Model file for the job. Use its own axes, mm. Face numbers are marked on the shaded views. A direction names the side the tool comes from. Give positions to 0.01 mm unless a question says otherwise; leave off trailing zeros. Write each loop counter-clockwise with the first axis right and the second up, starting at its lowest first coordinate (ties: lowest second). Pieces come first, ordered by that corner, then holes. Notation, with made-up numbers: (-29.75, 26.5) - (14.25, 26.5) arc R16 cw to (14.25, 33.5) - close; hole circle Ø11 at (-1.5, 85). An arc over 180 degrees is marked (long way). One line per item, written item: value. Start each with the question number.
(1) Cut at A-A, the plane y = -1.25. List the corners of the cut face in (x, z).
(2) Cut at D-D, the plane x = 0. List the corners of the cut face in (y, z), and give its area (3 significant figures).
(3) Cut at B-B, the plane x = 3.25. List the corners of the cut face in (y, z).
(4) Probe L1, parallel to X at y = 0.25, z = 0.45; L2, parallel to Y at x = -3.5, z = 0.25; L3, parallel to X at y = -1.75, z = 0.5. List the from-to ranges inside material, lowest first.
(5) 3-axis set-ups, long thin cutter, end or side, ignore diameter. For the marked faces 1, 2 and 3: which of +Z, -Z, +X, -X, +Y, -Y reach the whole face in a straight line?
(6) Cut at C-C, the plane z = 0.15. List the corners of the cut face in (x, y), and give its area (3 significant figures).
(7) Drop a flat-ended pin along its axis: P1, Ø2, axis at x = -0.5, y = -3, coming from the -Z side. Give the stop position or say it passes through.
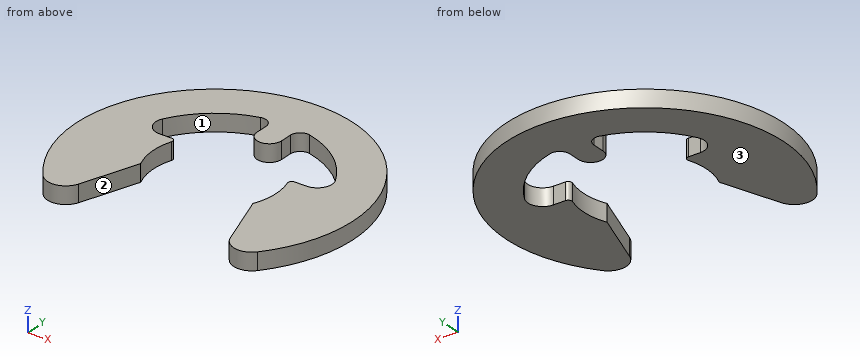
Autodesk Inventor part; units mm, degrees
ref_plane "Work Plane1" through (0, -2.9764, 0) normal (-1, 0, 0) x (0, 0, 1)
ref_plane "YZ Plane" through (0, 0, 0) normal (1, 0, 0) x (0, 1, 0)
ref_plane "XZ Plane" through (0, 0, 0) normal (0, 1, 0) x (-1, 0, 0)
sketch "Sketch1" plane through (0, 0, 0) normal (0, 0, 1) x (1, 0, 0)
  circle A0 centre (0, -2.9764) radius 3 construction
  line L0 (-0.5, 0.0236) -> (0, 0.0236) construction
  line L1 (-3.206, 0) -> (3.4858, 0)
  line L2 (-2.2913, -3.9764) -> (2.2913, -3.9764) construction
  arc A1 (-2.3679, -2.1745) -> (-2.2913, -3.9764) centre (0, -2.9764) ccw
  line L3 (0, 1.949) -> (0, -3.4788)
  arc A2 (-0.5, 0.0236) -> (0.5, 0.0236) centre (0, 0.0236) ccw
  arc A3 (4.3864, -6.5375) -> (-4.3864, -6.5375) centre (0, -2.9764) ccw
  line L4 (-3, -1.9764) -> (-2.51, -1.9764)
  line L5 (-0.5, 0.0236) -> (-0.5, 0.5093)
  arc A4 (-1, 0.8966) -> (-3.5294, -1.094) centre (0, -2.9764) ccw
  arc A5 (-0.5, 0.5093) -> (-1, 0.8966) centre (-0.9, 0.5093) ccw
  arc A6 (-3.5294, -1.094) -> (-3, -1.9764) centre (-3, -1.3764) ccw
  arc A7 (-2.3679, -2.1745) -> (-2.51, -1.9764) centre (-2.51, -2.1264) ccw
  line L6 (0, 2.6736) -> (2.5298, 2.6736) construction
  line L7 (-2.2913, -3.9764) -> (-3.0951, -6.3091)
  arc A8 (-4.3864, -6.5375) -> (-3.0951, -6.3091) centre (-3.8041, -6.0648) ccw
  line L8 (0, -0.4764) -> (-1.2778, -0.4764) construction
  line L9 (2.2913, -3.9764) -> (3.0951, -6.3091)
  arc A9 (3.0951, -6.3091) -> (4.3864, -6.5375) centre (3.8041, -6.0648) ccw
  arc A10 (2.2913, -3.9764) -> (2.3679, -2.1745) centre (0, -2.9764) ccw
  line L10 (3, -1.9764) -> (2.51, -1.9764)
  line L11 (0.5, 0.0236) -> (0.5, 0.5093)
  arc A11 (3.5294, -1.094) -> (1, 0.8966) centre (0, -2.9764) ccw
  arc A12 (1, 0.8966) -> (0.5, 0.5093) centre (0.9, 0.5093) ccw
  arc A13 (3, -1.9764) -> (3.5294, -1.094) centre (3, -1.3764) ccw
  arc A14 (2.51, -1.9764) -> (2.3679, -2.1745) centre (2.51, -2.1264) ccw
  point P0 (0.5, 0.0236)
  dimension "d0" = 6
  dimension "d3" = 1
  dimension "d4" = 0.5
  dimension "d5" = 11.3
  dimension "d8" = 4
  dimension "d9" = 1
  dimension "d10" = 0.4
  dimension "d11" = 0.6
  dimension "d12" = 0.15
  dimension "d13" = 0.75
  dimension "d14" = 2.5
  dimension "d15" = 2.5
extrude "Body" add sketch "Sketch1" along normal blind 0.7 contours A4 A6 L4 A7 A1 L7 A8 A3 A9 L9 A10 A14 L10 A13 A11 A12 L11 A2 L1 L5 A5 | L1 L3 A2 | L1 A2 L3
ref_plane "Work Plane1" through (0, -2.9764, 0) normal (-1, 0, 0) x (0, 0, 1)
equation "\"d0\" = WD"
equation "\"d3\" = 0.2 * ND"
equation "\"d4\" = 0.1 * ND"
equation "\"d5\" = SD2"
equation "\"d8\" = 0.8 * ND"
equation "\"d9\" = 0.2 * ND"
equation "\"d10\" = 0.08 * ND"
equation "\"d11\" = 0.12 * ND"
equation "\"d12\" = 0.03 * ND"
equation "\"d13\" = 0.15 * ND"
equation "\"d14\" = 0.5 * ND"
equation "\"d15\" = 0.5 * ND"
equation "\"d16\" = SD"
equation "\"ND\" = 5"
equation "\"SD\" = 0.7"
equation "\"WD\" = 6"
equation "\"d1\" = 1.6 * ND"
equation "\"d2\" = ND"
equation "\"SD2\" = 11.3"
equation "\"d6\" = ND"
equation "\"d7\" = 0.15 * ND"
equation "\"WDMIN\" = 5"
equation "\"SNB\" = 0.74"
equation "\"WDMAX\" = 7"
equation "\"BUBRMI\" = 1.2"
properties part number "DIN 6799 - 5" material "Steel, Mild"
Answers follow:
1. outline: (-5.38, 0) - (-3.59, 0) - (-3.59, 0.7) - (-5.38, 0.7) - close; (3.59, 0) - (5.38, 0) - (5.38, 0.7) - (3.59, 0.7) - close
2. outline: (-0.48, 0) - (2.67, 0) - (2.67, 0.7) - (-0.48, 0.7) - close
2. area: 2.20 mm²
3. outline: (-6.57, 0) - (-1.92, 0) - (-1.92, 0.7) - (-6.57, 0.7) - close; (-0.64, 0) - (1.65, 0) - (1.65, 0.7) - (-0.64, 0.7) - close
4. L1: x = -4.64 to -2.36, -0.5 to 0.5, 2.36 to 4.64
4. L2: y = -6.75 to -1.71, -1.04 to 1.46
4. L3: x = -5.52 to -3.47, 3.47 to 5.52
5. face 1: +Z, -Z
5. face 2: +Z, -Z, -Y
5. face 3: -Z, +X, -X, +Y, -Y
6. outline: (-4.39, -6.54) arc R0.75 ccw to (-3.1, -6.31) - (-2.29, -3.98) arc R2.5 cw to (-2.37, -2.17) arc R0.15 ccw to (-2.51, -1.98) - (-3, -1.98) arc R0.6 cw to (-3.53, -1.09) arc R4 cw to (-1, 0.9) arc R0.4 cw to (-0.5, 0.51) - (-0.5, 0.02) arc R0.5 ccw to (0.5, 0.02) - (0.5, 0.51) arc R0.4 cw to (1, 0.9) arc R4 cw to (3.53, -1.09) arc R0.6 cw to (3, -1.98) - (2.51, -1.98) arc R0.15 ccw to (2.37, -2.17) arc R2.5 cw to (2.29, -3.98) - (3.1, -6.31) arc R0.75 ccw to (4.39, -6.54) arc R5.65 ccw (long way) to start
6. area: 48.9 mm²
7. P1: passes through
